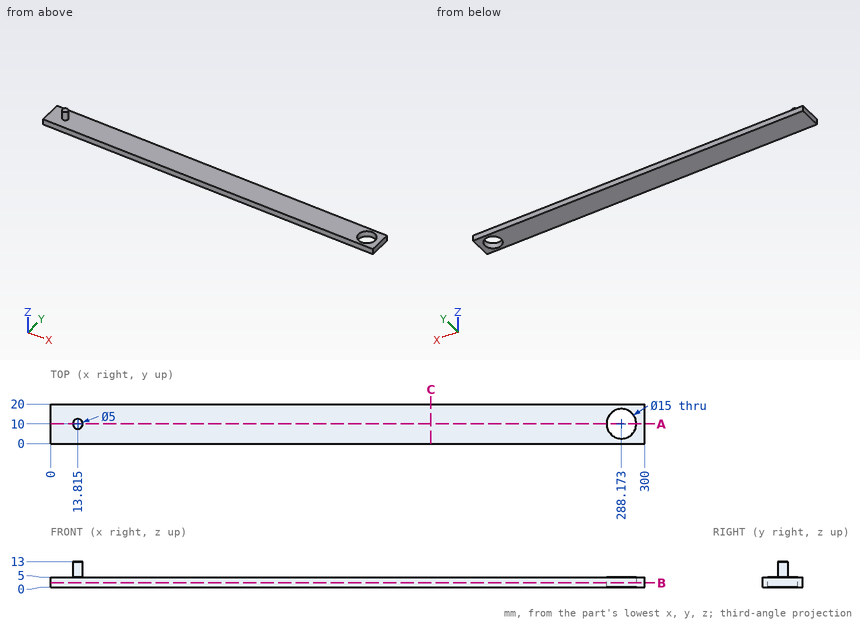
Can you work these out from the drawing? Everything is in mm from the part's minimum corner. Round coordinates to 2 decimals unless told otherwise and drop trailing zeros. Loops run counter-clockwise (first coordinate to the right, second up) from the corner with the lowest first, then second, coordinate; pieces in that order, holes last. Notation, with made-up numbers: (65.25, -24) - (101.25, -24) arc R21 cw to (101.25, -13) - close; hole circle Ø2 at (82.5, 15). An arc over 180 degrees is marked (long way). One line per question, with ' | ' between items. Start each with the question number.
Q1. I want a section at C-C (x = 192). Write out the boundary of the cut face in (y, z), then the cut area to 3 significant figures.
Q2. Will these pins go through, and if not, where does the flat tip stop? pin 1 (1 mm diameter, centred on x = 115, z = 7, fed in from +Y); pin 2 (10 mm diameter, centred on x = 201, y = 9, fed in from +Z).
Q3. Please list where these lines run through material, in increasing order: line 1 (X direction, y = 9.75, z = 2.75); line 2 (Z direction, x = 14, y = 6.25); line 3 (X direction, y = 8.5, z = 3). Write a range as [from, to].
Q4. I want a section at A-A (y = 10). Write out the boundary of the cut face in (x, z) (3 decimals), then the cut area to 4 significant figures.
Q5. I want a section at B-B (z = 2.25). Write out the boundary of the cut face in (x, y), then the cut area to 3 significant figures.
Response values:
1) outline: (0, 0) - (20, 0) - (20, 5) - (0, 5) - close | area: 100 mm²
2) pin 1: passes through | pin 2: stops at z = 5
3) line 1: x = [0, 280.68], [295.67, 300] | line 2: z = [0, 5] | line 3: x = [0, 280.82], [295.52, 300]
4) outline: (0, 0) - (280.673, 0) - (280.673, 5) - (16.315, 5) - (16.315, 13) - (11.315, 13) - (11.315, 5) - (0, 5) - close; (295.673, 0) - (300, 0) - (300, 5) - (295.673, 5) - close | area: 1,465 mm²
5) outline: (0, 0) - (300, 0) - (300, 20) - (0, 20) - close; hole circle Ø15 at (288.17, 10) | area: 5,820 mm²
